Could you check a few things on this model? Use its own coordinates, in mm. A direction names the side the tool comes from. Give positions to 0.01 mm unless a question says otherwise; leave off trailing zeros. Loops run counter-clockwise (first coordinate to the right, second up) from the corner with the lowest first, then second, coordinate; pieces in that order, holes last. Notation, with made-up numbers: (30.5, -16) - (83.5, -16) arc R19 ccw to (83.5, -12) - close; hole circle Ø6 at (5, 71.25). An arc over 180 degrees is marked (long way). One line per item, written item: value. Start each with the question number.
Q1. I want a section at B-B (y = 8). Please give me the cut outline in (x, z), then the cut area to 3 significant figures.
Q2. For faces 4 (the face through (30, -7, -18)), 5 (the face through (33, 21, 4)), 6 (the face through (38, 27, 0)), 7 (the face through (-27.092, -7.395, 9.399)), which set-ups out of +Z, -Z, +X, -X, +Y, -Y let a thin tool reach every point of the face, with its end or its side?
Q3. I want a section at A-A (z = 38.5). Please give me the cut outline in (x, y), then the cut area to 3 significant figures.
Q4. If I drill on line 1 (X direction, y = -5, z = 29); line 2 (X direction, y = -10, z = 10); line 3 (Y direction, x = 33.5, z = 34), over which ranges is the centre line in solid material (lowest first)? Write a range as from..to.
Q5. I want a section at D-D (y = 52). Please give me the cut outline in (x, z), then the cut area to 3 significant figures.
Q6. I want a section at C-C (z = 0). Please give me the cut outline in (x, y).
Q7. I'm going to push flat-ended pins straight in: P1, Ø6, axis at x = 6, y = 48, coming from the -Z side; P2, Ø2, axis at x = -22, y = 75, coming from the +Z side; P3, Ø3, axis at x = -10, z = 29, coming from the +Y side; P4, Ø7, axis at x = 35, z = 1.5, coming from the -Y side. Where does each tip first touch, or does it pass through?
Q8. If we mould it in two halves opening along Y, with no side actions, what happens to faces 1 (the face through (36, 0, -1)), 2 (the face through (-28.974, 15.776, -1.219)), 3 (the face through (-10, -7, 31))? For each: released by +Y, released by -Y, zero draft, split by the parting line, or undercut.
```python
from build123d import *

# Parameters (mm, degrees)
SKETCH1_R           = 29
BOSS_EXTRUDE1_DEPTH = 32
SKETCH3_W           = 8
SKETCH3_H           = 82.55
BOSS_EXTRUDE2_DEPTH = 38
SKETCH5_W           = 58
SKETCH5_H           = 15
BOSS_EXTRUDE3_DEPTH = 30
BOSS_EXTRUDE4_DEPTH = 15
SKETCH7_R           = 2
CUT_EXTRUDE2_DEPTH  = 16


with BuildPart() as part:
    # Sketch1 → Boss-Extrude1 (new body)
    with BuildSketch(Plane(origin=(0, 0, 0), x_dir=(1, 0, 0), z_dir=(0, 1, 0))):
        Circle(SKETCH1_R)
    extrude(amount=BOSS_EXTRUDE1_DEPTH)

    # Sketch2 → Revolve1 (revolve)
    with BuildSketch(Plane.XY):
        with BuildLine():
            Line((-29, 32), (0, 32))
            Line((0, 32), (0, 106))
            ThreePointArc((0, 106), (-35.617387288, 84.204442392), (-32.419733751, 42.570086139))
            ThreePointArc((-32.419733751, 42.570086139), (-29.876205733, 37.554756969), (-29, 32))
        make_face()
    revolve(axis=Axis((0, 32, 0), (0, 1, 0)))

    # Sketch3 → Boss-Extrude2 (add)
    with BuildSketch(Plane(origin=(0, 0, 0), x_dir=(0, 0, -1), z_dir=(1, 0, 0))):
        with Locations((0, 41.275)):
            Rectangle(SKETCH3_W, SKETCH3_H)
    extrude(amount=BOSS_EXTRUDE2_DEPTH)

    # Sketch5 → Boss-Extrude3 (add, symmetric)
    with BuildSketch(Plane(origin=(0, 0, 0), x_dir=(0, 0, -1), z_dir=(1, 0, 0))):
        with Locations((0, -7.5)):
            Rectangle(SKETCH5_W, SKETCH5_H)
    extrude(amount=BOSS_EXTRUDE3_DEPTH, both=True)

    # Sketch6 → Boss-Extrude4 (add)
    with BuildSketch(Plane.XZ.offset(15)):
        with BuildLine():
            Line((-37, -43), (-43, -43))
            Line((-43, -43), (-43, 43))
            Line((-43, 43), (43, 43))
            Line((43, 43), (43, 37))
            ThreePointArc((43, 37), (19.568542495, -19.568542495), (-37, -43))
        make_face()
    extrude(amount=-BOSS_EXTRUDE4_DEPTH)

    # Sketch7 → Cut-Extrude2 (cut, through all)
    with BuildSketch(Plane(origin=(0, 0, 0), x_dir=(1, 0, 0), z_dir=(0, 1, 0))):
        with Locations((-29, -10)):
            Circle(SKETCH7_R)
        with Locations((-10, -29)):
            Circle(SKETCH7_R)
    extrude(amount=-CUT_EXTRUDE2_DEPTH, mode=Mode.SUBTRACT)


solid = part.part
```
Worked answers:
1. outline: (28.72, -4) - (38, -4) - (38, 4) - (28.72, 4) arc R29 ccw (long way) to start
1. area: 2,710 mm²
2. face 4: -Z, +X, -Y
2. face 5: +Z, +X
2. face 6: +Z, -Z, +X, -Y
2. face 7: -Y
3. outline: (-43, -15) - (43, -15) - (43, 0) - (-43, 0) - close; circle Ø21.7 at (0, 66)
3. area: 1,660 mm²
4. line 1: x = -43..-12, -8..42.6
4. line 2: x = -43..-31, -27..38.31
4. line 3: y = -15..0
5. outline: (37.26, -4) - (38, -4) - (38, 4) - (37.26, 4) arc R37.47 ccw (long way) to start
5. area: 4,420 mm²
6. outline: (-43, -15) - (33.93, -15) - (33.93, 0) - (38, 0) - (38, 53.51) arc R40 ccw to (38, 78.49) - (38, 82.55) - (36.42, 82.55) arc R40 ccw (long way) to (-32.42, 42.57) arc R18.05 cw to (-29, 32) - (-29, 0) - (-43, 0) - close
7. P1: stops at z = -36.67
7. P2: stops at z = 32.89
7. P3: stops at y = 93.36
7. P4: stops at y = -15
8. face 1: released by -Y
8. face 2: undercut
8. face 3: zero draft
